from build123d import *

# Parameters (mm, degrees)
SKETCH1_W                 = 42
SKETCH1_H                 = 127
BOSS_EXTRUDE1_DEPTH       = 5.1
SKETCH2_W                 = 40
SKETCH2_H                 = 6
CUT_EXTRUDE1_DEPTH        = 8.2
SKETCH3_W                 = 15
SKETCH3_H                 = 2
BOSS_EXTRUDE2_DEPTH       = 1
TAB_PROFILE_W             = 10.5
TAB_PROFILE_H             = 1
F_6_CLEARANCE_HOLE1_D     = 3.6576
F_6_CLEARANCE_HOLE1_DEPTH = 1
F_6_CLEARANCE_HOLE2_D     = 3.6576
F_6_CLEARANCE_HOLE2_DEPTH = 1


with BuildPart() as part:
    # Sketch1 → Boss-Extrude1 (new, symmetric)
    with BuildSketch(Plane.XY):
        with Locations((0, 63.5)):
            Rectangle(SKETCH1_W, SKETCH1_H)
    extrude(amount=BOSS_EXTRUDE1_DEPTH, both=True)

    # Sketch2 → Cut-Extrude1 (cut)
    with BuildSketch(Plane.XY.offset(5.1)):
        with Locations((0, 124)):
            Rectangle(SKETCH2_W, SKETCH2_H)
    extrude(amount=-CUT_EXTRUDE1_DEPTH, mode=Mode.SUBTRACT)

    # Sketch3 → Boss-Extrude2 (add, symmetric)
    with BuildSketch(Plane(origin=(0, 0, -4.1), x_dir=(-1, 0, 0), z_dir=(0, 0, -1))):
        with Locations((-10.5, 128)):
            Rectangle(SKETCH3_W, SKETCH3_H)
        with Locations((10.5, 128)):
            Rectangle(SKETCH3_W, SKETCH3_H)
    extrude(amount=BOSS_EXTRUDE2_DEPTH, both=True)

    # Tabs: sweep along a path in Tab Bend
    with BuildLine(Plane(origin=(0, 0, 0), x_dir=(0, 0, -1), z_dir=(1, 0, 0))) as tabs_path:
        Line((4.1, 129), (4.1, 134))
        ThreePointArc((4.1, 134), (3.807106781, 134.707106781), (3.1, 135))
        Line((3.1, 135), (-3.1, 135))
    # Tab Profile → Tabs (sweep)
    with BuildSketch(Plane(origin=(0, 129, 0), x_dir=(1, 0, 0), z_dir=(0, 1, 0))):
        with Locations((-10.5, 4.1)):
            Rectangle(TAB_PROFILE_W, TAB_PROFILE_H)
        with Locations((10.5, 4.1)):
            Rectangle(TAB_PROFILE_W, TAB_PROFILE_H)
    sweep(path=tabs_path.line)

    # #6 Clearance Hole1
    with Locations(Plane(origin=(0, 135.5, 0), x_dir=(1, 0, 0), z_dir=(0, 1, 0))):
        with Locations((-10.5, 0)):
            Hole(F_6_CLEARANCE_HOLE1_D / 2, depth=F_6_CLEARANCE_HOLE1_DEPTH)

    # #6 Clearance Hole2
    with Locations(Plane(origin=(0, 135.5, 0), x_dir=(1, 0, 0), z_dir=(0, 1, 0))):
        with Locations((10.5, 0)):
            Hole(F_6_CLEARANCE_HOLE2_D / 2, depth=F_6_CLEARANCE_HOLE2_DEPTH)


solid = part.part
Verification items for the finished model (mm, model axes). A direction names the side the tool comes from. Round coordinates to 2 decimals unless told otherwise and drop trailing zeros. Write each loop counter-clockwise with the first axis right and the second up, starting at its lowest first coordinate (ties: lowest second). Pieces come first, ordered by that corner, then holes.
(1) Depth check by flat-ended pin: pin 1 Ø2 at (x, z) = (-12.5, -4.5) entering from +Y; pin 2 Ø4 at (x, y) = (-7, 123.5) entering from +Z; pin 3 Ø1.1 at (x, y) = (-12.5, 135) entering from +Z. Enter the tip coordinate at first touch or a pass-through.
Returned:
pin 1: stops at y = 135.45
pin 2: stops at z = -3.1
pin 3: stops at z = 3.1
(2) Mould release check, pull along Y, two halves, no side actions. Record for faces 6 (the flat face through (10, 134.5, 2)), 7 (the flat face through (11, 135.5, 2)), 8 (the flat face through (20, 124, 1)): pulls with the +Y half, pulls with the -Y half, needs draft (parallel to the pull), parting line crosses it, or undercut.
Returned:
face 6: undercut
face 7: pulls with the +Y half
face 8: needs draft
(3) Section check A-A (x = -10.5). Enter the section's corners in (y, z), plus the area to 3 significant figures.
Returned:
outline: (0, -5.1) - (129, -5.1) - (129, -4.6) - (134, -4.6) arc R1.5 ccw to (135.5, -3.1) - (135.5, -1.83) - (134.5, -1.83) - (134.5, -3.1) arc R0.5 cw to (134, -3.6) - (129, -3.6) - (129, -3.1) - (121, -3.1) - (121, 5.1) - (0, 5.1) - close; (134.5, 1.83) - (135.5, 1.83) - (135.5, 3.1) - (134.5, 3.1) - close
area: 1,260 mm2
(4) Section check B-B (z = 0). Enter the section's corners in (x, y).
Returned:
outline: (-21, 0) - (21, 0) - (21, 127) - (20, 127) - (20, 121) - (-20, 121) - (-20, 127) - (-21, 127) - close; (-15.75, 134.5) - (-12.33, 134.5) - (-12.33, 135.5) - (-15.75, 135.5) - close; (-8.67, 134.5) - (-5.25, 134.5) - (-5.25, 135.5) - (-8.67, 135.5) - close; (5.25, 134.5) - (8.67, 134.5) - (8.67, 135.5) - (5.25, 135.5) - close; (12.33, 134.5) - (15.75, 134.5) - (15.75, 135.5) - (12.33, 135.5) - close
(5) Material ranges on line 1 (Y direction, x = 7, z = -1.5); line 2 (Y direction, x = -3.5, z = 0.5); line 3 (Z direction, x = -10, y = 135), recorded low to high.
Returned:
line 1: y = 0 to 121, 134.5 to 135.5
line 2: y = 0 to 121
line 3: z = -4.22 to -1.76, 1.76 to 3.1
(6) Section check C-C (x = 0.5). Enter the section's corners in (y, z), plus the area to 3 significant figures.
Returned:
outline: (0, -5.1) - (127, -5.1) - (127, -3.1) - (121, -3.1) - (121, 5.1) - (0, 5.1) - close
area: 1,250 mm2
(7) Access from +Z, -Z, +X, -X, +Y, -Y to the whole of each face (thin tool, end or side, straight path). Record for faces 1 (the flat face through (11, 132, -4.6)), 2 (the flat face through (15.75, 135, -2)), 3 (the flat face through (10, 132, -3.6)), 4 (the cylindrical face through (-9.049, 134.993, 1.113)), 5 (the flat face through (-20, 124, 1)).
Returned:
face 1: -Z, +X, -X, +Y
face 2: +Z, -Z, +X, +Y
face 3: +Z, +X, -X
face 4: +Y
face 5: +Z, +Y
